Can you work these out from the model? Positions are in its coordinate system, mm. A direction names the side the tool comes from. Give positions to 0.01 mm unless a question says otherwise; leave off trailing zeros. Loops run counter-clockwise (first coordinate to the right, second up) from the corner with the lowest first, then second, coordinate; pieces in that order, holes last. Notation, with made-up numbers: (71.5, 6) - (79.5, 6) arc R18 ccw to (79.5, 31) - close; hole circle Ø2 at (44, 21.5). An arc over 180 degrees is marked (long way). Answer as a JSON object with one key per item and string values.
```python
from build123d import *

# Parameters (mm, degrees)
SKETCH1_R           = 5.926666667
BOSS_EXTRUDE1_DEPTH = 22.552
BOSS_EXTRUDE2_DEPTH = 3.386666667


with BuildPart() as part:
    # Sketch1 → Boss-Extrude1 (new body)
    with BuildSketch(Plane.XY):
        with Locations((-166.361835023, 44.902323519)):
            Circle(SKETCH1_R)
    extrude(amount=BOSS_EXTRUDE1_DEPTH)

    # Sketch2 → Boss-Extrude2 (add)
    with BuildSketch(Plane.XY.offset(22.552)):
        with BuildLine():
            Line((-171.494478916, 41.938990186), (-166.361835023, 41.938990186))
            Line((-166.361835023, 41.938990186), (-161.22919113, 41.938990186))
            ThreePointArc((-161.22919113, 41.938990186), (-160.637114626, 43.368389312), (-160.435168356, 44.902323519))
            ThreePointArc((-160.435168356, 44.902323519), (-167.89576923, 50.627043916), (-171.494478916, 41.938990186))
        make_face()
    extrude(amount=BOSS_EXTRUDE2_DEPTH)


solid = part.part
```
1) Which directions (+Z, -Z, +X, -X, +Y, -Y) give clear straight access to the entire face, cutting with the end or side of a thin tool? Please do faces 1 (the flat face through (-166, 41.939, 24)), 2 (the flat face through (-166, 45, 0)).
Check sheet entries:
{"face 1": "+Z, +X, -X, -Y", "face 2": "-Z, +X, -X, +Y, -Y"}
2) I'm going to push flat-ended pins straight in: P1, Ø1.5, axis at y = 48.5, z = 14, coming from the -X side; P2, Ø4, axis at x = -163.5, z = 4, coming from the -Y side; P3, Ø0.9, axis at x = -169, y = 40.5, coming from the +Z side. Where does each tip first touch, or does it pass through?
Check sheet entries:
{"P1": "x = -171.56", "P2": "y = 39.04", "P3": "z = 22.55"}
3) I need wall thicknesses on L1, parallel to Y at x = -165, z = 11; L2, parallel to Y at x = -170.5, z = 9.25; L3, parallel to X at y = 45.5, z = 24.5. Which ranges of each line are inside material? Lowest first, please.
Check sheet entries:
{"L1": "39.13 to 50.67", "L2": "40.66 to 49.15", "L3": "-172.26 to -160.47"}
4) Imagine slicing it at B-B on y = 47.5. Write out the boundary of the cut face in (x, z), and give its area (3 significant figures).
Check sheet entries:
{"outline": "(-171.69, 0) - (-161.03, 0) - (-161.03, 25.94) - (-171.69, 25.94) - close", "area": "276 mm2"}
5) Imagine slicing it at D-D on x = -168.75. Write out the boundary of the cut face in (y, z).
Check sheet entries:
{"outline": "(39.48, 0) - (50.33, 0) - (50.33, 25.94) - (41.94, 25.94) - (41.94, 22.55) - (39.48, 22.55) - close"}
6) Imagine slicing it at C-C on z = 23. Write out the boundary of the cut face in (x, y), and give its area (3 significant figures).
Check sheet entries:
{"outline": "(-171.49, 41.94) - (-161.23, 41.94) arc R5.93 ccw (long way) to start", "area": "88.8 mm2"}
7) Imagine slicing it at A-A on x = -165. Write out the boundary of the cut face in (y, z).
Check sheet entries:
{"outline": "(39.13, 0) - (50.67, 0) - (50.67, 25.94) - (41.94, 25.94) - (41.94, 22.55) - (39.13, 22.55) - close"}
